```python
from build123d import *

# Parameters (mm, degrees)
SKETCH2_W            = 100
SKETCH2_H            = 100
BOSS_EXTRUDE1_DEPTH  = 5
SKETCH3_W            = 100
SKETCH3_H            = 100
BOSS_EXTRUDE2_DEPTH  = 5
SKETCH8_R            = 5
BOSS_EXTRUDE7_DEPTH  = 30
BOSS_EXTRUDE21_DEPTH = 10
FILLET14_R           = 4
FILLET13_R           = 4
SKETCH24_W           = 10
SKETCH24_H           = 10
BOSS_EXTRUDE22_DEPTH = 15
BOSS_EXTRUDE25_DEPTH = 10
SKETCH26_W           = 10
SKETCH26_H           = 10
BOSS_EXTRUDE26_DEPTH = 15
FILLET18_R           = 4
FILLET17_R           = 4
BOSS_EXTRUDE23_DEPTH = 10
SKETCH25_W           = 10
SKETCH25_H           = 10
BOSS_EXTRUDE24_DEPTH = 15
FILLET15_R           = 4
FILLET16_R           = 4
BOSS_EXTRUDE10_DEPTH = 10
FILLET19_R           = 4
SKETCH27_W           = 10
SKETCH27_H           = 10
BOSS_EXTRUDE27_DEPTH = 15
FILLET20_R           = 4
SKETCH62_R           = 11.223510807
CUT_EXTRUDE3_DEPTH   = 30
SKETCH64_W           = 35.4
SKETCH64_H           = 35.4
BOSS_EXTRUDE53_DEPTH = 25.4
SKETCH66_W           = 25.4
SKETCH66_H           = 25.4
CUT_EXTRUDE4_DEPTH   = 12.7
SKETCH67_W           = 50
SKETCH67_H           = 50
BOSS_EXTRUDE54_DEPTH = 5
SKETCH68_W           = 17.3
SKETCH68_H           = 10
BOSS_EXTRUDE55_DEPTH = 10
SKETCH70_W           = 17.3
SKETCH70_H           = 10
BOSS_EXTRUDE57_DEPTH = 10
SKETCH74_W           = 17.3
SKETCH74_H           = 10
BOSS_EXTRUDE58_DEPTH = 10
BOSS_EXTRUDE59_DEPTH = 10
BOSS_EXTRUDE60_DEPTH = 10
BOSS_EXTRUDE61_DEPTH = 10
BOSS_EXTRUDE62_DEPTH = 10
BOSS_EXTRUDE63_DEPTH = 10
BOSS_EXTRUDE64_DEPTH = 10
SKETCH85_W           = 17.3
SKETCH85_H           = 10
BOSS_EXTRUDE65_DEPTH = 10
BOSS_EXTRUDE66_DEPTH = 10
BOSS_EXTRUDE67_DEPTH = 10


with BuildPart() as part:
    # Sketch2 → Boss-Extrude1 (new body)
    with BuildSketch(Plane(origin=(0, 0, 0), x_dir=(1, 0, 0), z_dir=(0, 1, 0))):
        Rectangle(SKETCH2_W, SKETCH2_H)
    extrude(amount=BOSS_EXTRUDE1_DEPTH)

    # Sketch3 → Boss-Extrude2 (add)
    with BuildSketch(Plane.XZ):
        Rectangle(SKETCH3_W, SKETCH3_H)
    extrude(amount=BOSS_EXTRUDE2_DEPTH)

    # Sketch8 → Boss-Extrude7 (add)
    with BuildSketch(Plane.XZ.offset(5)):
        with Locations(Location((0, 0, 0), (0, 0, 90))):
            Circle(SKETCH8_R)
    extrude(amount=BOSS_EXTRUDE7_DEPTH)

    # Sketch11 → Boss-Extrude21 (add)
    with BuildSketch(Plane(origin=(50, 0, 0), x_dir=(0, 0, -1), z_dir=(1, 0, 0))):
        Polygon((5, -5), (5, 12.5), (1, 12.5), (1, 9.5), (3, 5), (-3, 5), (-1, 9.5), (-1, 12.5), (-5, 12.5), (-5, -5), align=None)
    extrude(amount=BOSS_EXTRUDE21_DEPTH)

    # Fillet14
    # the kernel refuses this fillet: 4 mm, written as the material it takes off along each edge
    with BuildSketch(Plane(origin=(40.317541634, 12.5, -1), x_dir=(0, -1, 0), z_dir=(1, 0, 0))) as fillet14_piece_1:
        with BuildLine():
            CenterArc((4, 3.872983346), FILLET14_R, 180, 75.522487814)
            Line((0, 3.872983346), (-0.08, 3.872983346))
            Line((-0.08, 3.872983346), (-0.08, 0))
            Line((-0.08, 0), (0, -0.08))
            ThreePointArc((0, -0.08), (1.5, -0.08), (2.98, -0.077459667))
            Line((2.98, -0.077459667), (3, 0))
        make_face()
    extrude(amount=29.364916731, mode=Mode.SUBTRACT)

    # Fillet13
    # the kernel refuses this fillet: 4 mm, written as the material it takes off along each edge
    with BuildSketch(Plane(origin=(40.317541634, 12.5, 1), x_dir=(0, 0, 1), z_dir=(1, 0, 0))) as fillet13_piece_1:
        with BuildLine():
            CenterArc((3.872983346, 4), FILLET13_R, 194.477512186, 75.522487814)
            Line((0, 3), (-0.077459667, 2.98))
            ThreePointArc((-0.077459667, 2.98), (-0.08, 1.5), (-0.08, 0))
            Line((-0.08, 0), (0, -0.08))
            Line((0, -0.08), (3.872983346, -0.08))
            Line((3.872983346, -0.08), (3.872983346, 0))
        make_face()
    extrude(amount=29.364916731, mode=Mode.SUBTRACT)

    # Sketch24 → Boss-Extrude22 (add)
    with BuildSketch(Plane(origin=(60, 0, 0), x_dir=(0, 0, -1), z_dir=(1, 0, 0))):
        Rectangle(SKETCH24_W, SKETCH24_H)
    extrude(amount=BOSS_EXTRUDE22_DEPTH)

    # Sketch13 → Boss-Extrude25 (add)
    with BuildSketch(Plane.ZY.offset(50)):
        Polygon((-5, 12.5), (-5, -5), (5, -5), (5, 12.5), (1, 12.5), (1, 9.5), (3, 5), (-3, 5), (-1, 9.5), (-1, 12.5), align=None)
    extrude(amount=BOSS_EXTRUDE25_DEPTH)

    # Sketch26 → Boss-Extrude26 (add)
    with BuildSketch(Plane.ZY.offset(60)):
        Rectangle(SKETCH26_W, SKETCH26_H)
    extrude(amount=BOSS_EXTRUDE26_DEPTH)

    # Fillet18
    # the kernel refuses this fillet: 4 mm, written as the material it takes off along each edge
    with BuildSketch(Plane(origin=(-40.317541634, 12.5, 1), x_dir=(0, -1, 0), z_dir=(-1, 0, 0))) as fillet18_piece_1:
        with BuildLine():
            CenterArc((4, 3.872983346), FILLET18_R, 180, 75.522487814)
            Line((0, 3.872983346), (-0.08, 3.872983346))
            Line((-0.08, 3.872983346), (-0.08, 0))
            Line((-0.08, 0), (0, -0.08))
            ThreePointArc((0, -0.08), (1.5, -0.08), (2.98, -0.077459667))
            Line((2.98, -0.077459667), (3, 0))
        make_face()
    extrude(amount=29.364916731, mode=Mode.SUBTRACT)

    # Fillet17
    # the kernel refuses this fillet: 4 mm, written as the material it takes off along each edge
    with BuildSketch(Plane(origin=(-40.317541634, 12.5, -1), x_dir=(0, 0, -1), z_dir=(-1, 0, 0))) as fillet17_piece_1:
        with BuildLine():
            CenterArc((3.872983346, 4), FILLET17_R, 194.477512186, 75.522487814)
            Line((0, 3), (-0.077459667, 2.98))
            ThreePointArc((-0.077459667, 2.98), (-0.08, 1.5), (-0.08, 0))
            Line((-0.08, 0), (0, -0.08))
            Line((0, -0.08), (3.872983346, -0.08))
            Line((3.872983346, -0.08), (3.872983346, 0))
        make_face()
    extrude(amount=29.364916731, mode=Mode.SUBTRACT)

    # Sketch14 → Boss-Extrude23 (add)
    with BuildSketch(Plane(origin=(0, 0, -50), x_dir=(-1, 0, 0), z_dir=(0, 0, -1))):
        Polygon((-5, 12.5), (-1, 12.5), (-1, 9.5), (-3, 5), (3, 5), (1, 9.5), (1, 12.5), (5, 12.5), (5, -5), (-5, -5), align=None)
    extrude(amount=BOSS_EXTRUDE23_DEPTH)

    # Sketch25 → Boss-Extrude24 (add)
    with BuildSketch(Plane(origin=(0, 0, -60), x_dir=(-1, 0, 0), z_dir=(0, 0, -1))):
        Rectangle(SKETCH25_W, SKETCH25_H)
    extrude(amount=BOSS_EXTRUDE24_DEPTH)

    # Fillet15
    # the kernel refuses this fillet: 4 mm, written as the material it takes off along each edge
    with BuildSketch(Plane(origin=(-1, 12.5, -40.317541634), x_dir=(0, -1, 0), z_dir=(0, 0, -1))) as fillet15_piece_1:
        with BuildLine():
            CenterArc((4, 3.872983346), FILLET15_R, 180, 75.522487814)
            Line((0, 3.872983346), (-0.08, 3.872983346))
            Line((-0.08, 3.872983346), (-0.08, 0))
            Line((-0.08, 0), (0, -0.08))
            ThreePointArc((0, -0.08), (1.5, -0.08), (2.98, -0.077459667))
            Line((2.98, -0.077459667), (3, 0))
        make_face()
    extrude(amount=29.364916731, mode=Mode.SUBTRACT)

    # Fillet16
    # the kernel refuses this fillet: 4 mm, written as the material it takes off along each edge
    with BuildSketch(Plane(origin=(1, 12.5, -40.317541634), x_dir=(0, -1, 0), z_dir=(0, 0, -1))) as fillet16_piece_1:
        with BuildLine():
            CenterArc((4, -3.872983346), FILLET16_R, 104.477512186, 75.522487814)
            Line((0, -3.872983346), (-0.08, -3.872983346))
            Line((-0.08, -3.872983346), (-0.08, 0))
            Line((-0.08, 0), (0, 0.08))
            ThreePointArc((0, 0.08), (1.5, 0.08), (2.98, 0.077459667))
            Line((2.98, 0.077459667), (3, 0))
        make_face()
    extrude(amount=29.364916731, mode=Mode.SUBTRACT)

    # Sketch12 → Boss-Extrude10 (add)
    with BuildSketch(Plane.XY.offset(50)):
        Polygon((-5, 12.5), (-5, -5), (5, -5), (5, 12.5), (1, 12.5), (1, 9.5), (3, 5), (-3, 5), (-1, 9.5), (-1, 12.5), align=None)
    extrude(amount=BOSS_EXTRUDE10_DEPTH)

    # Fillet19
    # the kernel refuses this fillet: 4 mm, written as the material it takes off along each edge
    with BuildSketch(Plane(origin=(-1, 12.5, 40.317541634), x_dir=(-1, 0, 0), z_dir=(0, 0, 1))) as fillet19_piece_1:
        with BuildLine():
            CenterArc((3.872983346, 4), FILLET19_R, 194.477512186, 75.522487814)
            Line((0, 3), (-0.077459667, 2.98))
            ThreePointArc((-0.077459667, 2.98), (-0.08, 1.5), (-0.08, 0))
            Line((-0.08, 0), (0, -0.08))
            Line((0, -0.08), (3.872983346, -0.08))
            Line((3.872983346, -0.08), (3.872983346, 0))
        make_face()
    extrude(amount=29.364916731, mode=Mode.SUBTRACT)

    # Sketch27 → Boss-Extrude27 (add)
    with BuildSketch(Plane.XY.offset(60)):
        Rectangle(SKETCH27_W, SKETCH27_H)
    extrude(amount=BOSS_EXTRUDE27_DEPTH)

    # Fillet20
    # the kernel refuses this fillet: 4 mm, written as the material it takes off along each edge
    with BuildSketch(Plane(origin=(1, 12.5, 40.317541634), x_dir=(1, 0, 0), z_dir=(0, 0, 1))) as fillet20_piece_1:
        with BuildLine():
            CenterArc((3.872983346, -4), FILLET20_R, 90, 75.522487814)
            Line((0, -3), (-0.077459667, -2.98))
            ThreePointArc((-0.077459667, -2.98), (-0.08, -1.5), (-0.08, 0))
            Line((-0.08, 0), (0, 0.08))
            Line((0, 0.08), (3.872983346, 0.08))
            Line((3.872983346, 0.08), (3.872983346, 0))
        make_face()
    extrude(amount=29.364916731, mode=Mode.SUBTRACT)

    # Sketch62 → Cut-Extrude3 (cut)
    with BuildSketch(Plane.XZ.offset(5)):
        Circle(SKETCH62_R)
    extrude(amount=CUT_EXTRUDE3_DEPTH, mode=Mode.SUBTRACT)

    # Sketch68 → Boss-Extrude55 (add)
    with BuildSketch(Plane.XY.offset(50)):
        with Locations((16.35, 0)):
            Rectangle(SKETCH68_W, SKETCH68_H)
    extrude(amount=BOSS_EXTRUDE55_DEPTH)

    # Sketch70 → Boss-Extrude57 (add)
    with BuildSketch(Plane(origin=(0, 0, -50), x_dir=(-1, 0, 0), z_dir=(0, 0, -1))):
        with Locations((16.35, 0)):
            Rectangle(SKETCH70_W, SKETCH70_H)
    extrude(amount=BOSS_EXTRUDE57_DEPTH)

    # Sketch74 → Boss-Extrude58 (add)
    with BuildSketch(Plane.ZY.offset(50)):
        with Locations((16.35, 0)):
            Rectangle(SKETCH74_W, SKETCH74_H)
    extrude(amount=BOSS_EXTRUDE58_DEPTH)



with BuildPart() as body_2:
    # Sketch64 → Boss-Extrude53 (new body)
    with BuildSketch(Plane(origin=(0, -72.5, 0), x_dir=(1, 0, 0), z_dir=(0, 1, 0))):
        Rectangle(SKETCH64_W, SKETCH64_H)
    extrude(amount=BOSS_EXTRUDE53_DEPTH)

    # Sketch66 → Cut-Extrude4 (cut)
    with BuildSketch(Plane(origin=(0, -72.5, 0), x_dir=(-1, 0, 0), z_dir=(0, -1, 0))):
        Rectangle(SKETCH66_W, SKETCH66_H)
    extrude(amount=-CUT_EXTRUDE4_DEPTH, mode=Mode.SUBTRACT)


with BuildPart() as body_3:
    # Sketch67 → Boss-Extrude54 (new body)
    with BuildSketch(Plane(origin=(0, 67.5, 0), x_dir=(1, 0, 0), z_dir=(0, 1, 0))):
        Rectangle(SKETCH67_W, SKETCH67_H)
    extrude(amount=-BOSS_EXTRUDE54_DEPTH)


with BuildPart() as part_1:
    add(part.part)

    add(body_2.part)  # Boss-Extrude59 merges body 2
    # Sketch76 → Boss-Extrude59 (add)
    with BuildSketch(Plane.ZY.offset(17.7)):
        Polygon((-17.7, -47.1), (-60, -5), (-50, -5), (-7.7, -47.1), align=None)
    extrude(amount=-BOSS_EXTRUDE59_DEPTH)


    add(body_3.part)  # Boss-Extrude60 merges body 3
    # Sketch77 → Boss-Extrude60 (add)
    with BuildSketch(Plane.ZY.offset(25)):
        Polygon((-25, 62.5), (-60, 5), (-50, 5), (-15, 62.5), align=None)
    extrude(amount=-BOSS_EXTRUDE60_DEPTH)

    # Sketch78 → Boss-Extrude61 (add)
    with BuildSketch(Plane.XY.offset(17.7)):
        Polygon((-17.7, -47.1), (-60, -5), (-50, -5), (-7.7, -47.1), align=None)
    extrude(amount=-BOSS_EXTRUDE61_DEPTH)

    # Sketch79 → Boss-Extrude62 (add)
    with BuildSketch(Plane.XY.offset(25)):
        Polygon((-25, 62.5), (-60, 5), (-50, 5), (-15, 62.5), align=None)
    extrude(amount=-BOSS_EXTRUDE62_DEPTH)

    # Sketch82 → Boss-Extrude63 (add)
    with BuildSketch(Plane(origin=(17.7, 0, 0), x_dir=(0, 0, -1), z_dir=(1, 0, 0))):
        Polygon((-60, -5), (-17.7, -47.1), (-7.7, -47.1), (-50, -5), align=None)
    extrude(amount=-BOSS_EXTRUDE63_DEPTH)

    # Sketch83 → Boss-Extrude64 (add)
    with BuildSketch(Plane(origin=(25, 0, 0), x_dir=(0, 0, -1), z_dir=(1, 0, 0))):
        Polygon((-25, 62.5), (-60, 5), (-50, 5), (-15, 62.5), align=None)
    extrude(amount=-BOSS_EXTRUDE64_DEPTH)

    # Sketch85 → Boss-Extrude65 (add)
    with BuildSketch(Plane(origin=(50, 0, 0), x_dir=(0, 0, -1), z_dir=(1, 0, 0))):
        with Locations((16.35, 0)):
            Rectangle(SKETCH85_W, SKETCH85_H)
    extrude(amount=BOSS_EXTRUDE65_DEPTH)

    # Sketch86 → Boss-Extrude66 (add)
    with BuildSketch(Plane(origin=(0, 0, -25), x_dir=(-1, 0, 0), z_dir=(0, 0, -1))):
        Polygon((-25, 62.5), (-60, 5), (-50, 5), (-15, 62.5), align=None)
    extrude(amount=-BOSS_EXTRUDE66_DEPTH)

    # Sketch89 → Boss-Extrude67 (add)
    with BuildSketch(Plane(origin=(0, 0, -17.7), x_dir=(-1, 0, 0), z_dir=(0, 0, -1))):
        Polygon((-60, -5), (-50, -5), (-7.7, -47.1), (-17.7, -47.1), align=None)
    extrude(amount=-BOSS_EXTRUDE67_DEPTH)


solid = part_1.part
```
The model under review builds one solid part; all positions refer to its coordinate system, in mm. A direction names the side the tool comes from. Give positions to 0.01 mm unless a question says otherwise; leave off trailing zeros. Write each loop counter-clockwise with the first axis right and the second up, starting at its lowest first coordinate (ties: lowest second). Pieces come first, ordered by that corner, then holes. Notation, with made-up numbers: (65, -38.75) -> (81, -38.75) arc R23 ccw to (81, -5.75) -> close; hole circle Ø10 at (54.5, 8.25). An arc over 180 degrees is marked (long way). Answer in a Markdown table with one row per item.
1) For L1, parallel to X at y = -64, z = 8.5; L2, parallel to Y at x = 33.5, z = 2.5; L3, parallel to X at y = 1.5, z = -58, list the stretches that pass through material, from the lowest coordinate up. Write a range as [from, to].
Worked answers:
| item | result |
|---|---|
| L1 | [-17.7, -12.7], [12.7, 17.7] |
| L2 | [-5, 5] |
| L3 | [-25, -7.7], [-5, 5] |
2) Add section D-D on z = 37.5. State the section outline as (x, y) points.
Worked answers:
| item | result |
|---|---|
| outline | (-50, -5) -> (50, -5) -> (50, 5) -> (-50, 5) -> close; (7.7, -27.39) -> (17.7, -27.39) -> (17.7, -17.44) -> (7.7, -17.44) -> close; (15, 25.54) -> (25, 25.54) -> (25, 41.96) -> (15, 41.96) -> close |
3) Add section A-A on x = -21.5. State the section outline as (y, z) points, plus the area to 3 significant figures.
Worked answers:
| item | result |
|---|---|
| outline | (-43.32, 7.7) -> (-33.37, 7.7) -> (-33.37, 17.7) -> (-43.32, 17.7) -> close; (-5, -60) -> (5, -60) -> (62.5, -25) -> (67.5, -25) -> (67.5, 25) -> (51.82, 25) -> (51.82, 15) -> (62.5, 15) -> (62.5, -15) -> (5, -50) -> (5, 50) -> (-5, 50) -> close |
| area | 2,130 mm² |
4) Mouldability with a two-part tool opening along Z and no side actions: class faces 1 (the flat face through (16, 0, 60)), 2 (the flat face through (25, 39, 30)), 3 (the cylindrical face through (-54.93, 11.64, -2.394)) as +Z half, -Z half, draft (parallel to the pull), parting line (faces both ways), or undercut.
Worked answers:
| item | result |
|---|---|
| face 1 | +Z half |
| face 2 | draft |
| face 3 | undercut |
5) Add section C-C on x = -44.5. State the section outline as (y, z) points.
Worked answers:
| item | result |
|---|---|
| outline | (-20.43, 7.7) -> (-10.47, 7.7) -> (-10.47, 17.7) -> (-20.43, 17.7) -> close; (-5, -50) -> (5, -50) -> (5, 50) -> (-5, 50) -> close; (14.04, 15) -> (30.46, 15) -> (30.46, 25) -> (14.04, 25) -> close |
6) Tool access review of faces 4 (the flat face through (-16, 0, -60)), 5 (the flat face through (37, 0, 50)), 6 (the flat face through (-50, 9, -3)), 7 (the flat face through (50, 9, -3)), 8 (the flat face through (12.7, -66, 0)): name each direction out of +Z, -Z, +X, -X, +Y, -Y from which nothing blocks a thin tool from reaching the whole face with its end or side.
Worked answers:
| item | result |
|---|---|
| face 4 | -Z, -X, +Y, -Y |
| face 5 | +Z, +X, +Y, -Y |
| face 6 | -Z, +Y |
| face 7 | +Z, +Y |
| face 8 | -Y |
7) Clearance check with flat-ended pins moving along their axes: P1, Ø5, axis at x = 31.5, y = 42, coming from the +Z side; P2, Ø9, axis at x = -64.5, y = 3.5, coming from the -Z side; P3, Ø2, axis at y = 9, z = 4, coming from the -X side. State where each tip first meets the part, or that it passes through.
Worked answers:
| item | result |
|---|---|
| P1 | z = -15 |
| P2 | z = -5 |
| P3 | x = -60 |
8) Add section B-B on y = 37. State the section outline as (x, z) points, plus the area to 3 significant figures.
Worked answers:
| item | result |
|---|---|
| outline | (-40.52, 15) -> (-30.52, 15) -> (-30.52, 25) -> (-40.52, 25) -> close; (-25, -40.52) -> (-15, -40.52) -> (-15, -30.52) -> (-25, -30.52) -> close; (15, 30.52) -> (25, 30.52) -> (25, 40.52) -> (15, 40.52) -> close; (30.52, -25) -> (40.52, -25) -> (40.52, -15) -> (30.52, -15) -> close |
| area | 400 mm² |
